Part model, mm, in its own coordinate system. Face numbers are marked on the shaded views. Round coordinates to 2 decimals unless told otherwise and drop trailing zeros. Write each loop counter-clockwise with the first axis right and the second up, starting at its lowest first coordinate (ties: lowest second). Pieces come first, ordered by that corner, then holes. Notation, with made-up numbers: M 13.5,58.25 L 42.5,58.25 A20 cw 42.5,74.25 Z; hole C 57.5,25.25 d7. An arc over 180 degrees is marked long. Use one line per item in the form item = value. Start each with the question number.
Item 1: Probe L1, parallel to X at y = 1.25, z = -4; L2, parallel to X at y = 1, z = -16; L3, parallel to X at y = 2.3, z = -13.25. List the from-to ranges inside material, lowest first.
Item 2: Cut at C-C, the plane z = -16.5. Give the cut face in (x, y).
Item 3: Cut at A-A, the plane x = 30. Give the cut face in (y, z), then the cut area to 3 significant figures.
Item 4: Cut at B-B, the plane z = -5.95. Give the cut face in (x, y).
Item 5: Cut at D-D, the plane y = 1.1. State how many separate pieces and enclosed holes the cut face has, then the cut area to 3 significant figures.
Item 6: Mould opens along Z. For the marked faces 1, 2 and 3 say: +Z half, -Z half, draft (parallel to the pull), parting line (faces both ways), or undercut.
Item 7: Flat gauge pins, fed straight in: pin 1 Ø1.5 at (x, y) = (31, 2) entering from +Z; pin 2 Ø0.9 at (y, z) = (2, -13) entering from -X; pin 3 Ø0.9 at (x, y) = (17, 1.5) entering from -Z; pin 4 Ø1 at (x, z) = (21.5, -1) entering from -Y. Where does each tip first touch, or does it go through?
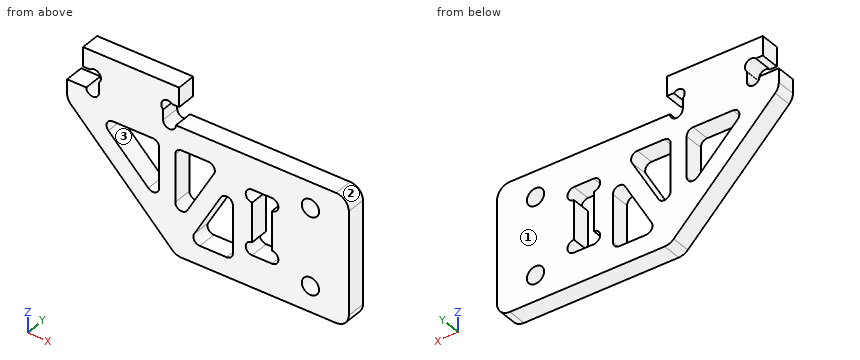
from build123d import *

# Parameters (mm, degrees)
EXTRUDE_1_DEPTH     = 3
SKETCH_2_R          = 1.35
SKETCH_2_W          = 3.1
SKETCH_2_H          = 10.1
CUT_EXTRUDE_1_DEPTH = 49.425200051
SKETCH_5_W          = 15
SKETCH_5_H          = 3
EXTRUDE_2_DEPTH     = 3
SKETCH_3_R          = 1
CUT_EXTRUDE_2_DEPTH = 49.425200051
CUT_EXTRUDE_3_DEPTH = 10
FILLET_1_R          = 1
FILLET_2_R          = 2


with BuildPart() as part:
    # 草图1 → 凸台-拉伸1 (new body)
    with BuildSketch(Plane(origin=(0, 0, 0), x_dir=(1, 0, 0), z_dir=(0, 1, 0))):
        Polygon((0, 0), (5, 0), (5, -3), (15, -3), (15, 0), (44, 0), (44, 20), (17, 20), (0, 3), align=None)
    extrude(amount=EXTRUDE_1_DEPTH)

    # 草图2 → 切除-拉伸1 (cut, through all)
    with BuildSketch(Plane.XZ):
        with Locations(Location((38, -16, 0), (0, 0, 270))):
            Circle(SKETCH_2_R)
        with Locations(Location((38, -4, 0), (0, 0, 90))):
            Circle(SKETCH_2_R)
        with Locations((30.45, -10)):
            Rectangle(SKETCH_2_W, SKETCH_2_H)
    extrude(amount=-CUT_EXTRUDE_1_DEPTH, mode=Mode.SUBTRACT)

    # 草图5 → 凸台-拉伸2 (add)
    with BuildSketch(Plane(origin=(0, 3, 0), x_dir=(1, 0, 0), z_dir=(0, 1, 0))):
        with Locations((10, -4.5)):
            Rectangle(SKETCH_5_W, SKETCH_5_H)
    extrude(amount=-EXTRUDE_2_DEPTH)

    # 草图3 → 切除-拉伸2 (cut, through all)
    with BuildSketch(Plane.XZ):
        with Locations((32, -14.05)):
            Circle(SKETCH_3_R)
        with Locations((16, 0)):
            Circle(SKETCH_3_R)
        with Locations((4, 0)):
            Circle(SKETCH_3_R)
        with Locations((32, -5.95)):
            Circle(SKETCH_3_R)
        with Locations((28.9, -5.95)):
            Circle(SKETCH_3_R)
        with Locations((28.9, -14.05)):
            Circle(SKETCH_3_R)
        with Locations((4.292893219, 2.292893219)):
            Circle(SKETCH_3_R)
        with Locations((15.707106781, 2.292893219)):
            Circle(SKETCH_3_R)
    extrude(amount=-CUT_EXTRUDE_2_DEPTH, mode=Mode.SUBTRACT)

    # 草图4 → 切除-拉伸3 (cut)
    with BuildSketch(Plane(origin=(0, 3, 0), x_dir=(1, 0, 0), z_dir=(0, 1, 0))):
        Polygon((23.789631314, 3.5), (16.896065397, 15.65342471), (16.896065397, 3.5), align=None)
        Polygon((14.396065397, 3.5), (14.396065397, 13.15342471), (4.742640687, 3.5), align=None)
        Polygon((25.9, 4.84657529), (25.9, 17), (19.006434083, 17), align=None)
    extrude(amount=-CUT_EXTRUDE_3_DEPTH, mode=Mode.SUBTRACT)

    # 圆角1
    fillet_1_edges = [part.edges().sort_by_distance(p)[0] for p in [
        (19.006434083, 1.5, -17),
        (25.9, 1.5, -17),
        (25.9, 1.5, -4.84657529),
        (14.396065397, 1.5, -13.15342471),
        (14.396065397, 1.5, -3.5),
        (4.742640687, 1.5, -3.5),
        (16.896065397, 1.5, -15.65342471),
        (23.789631314, 1.5, -3.5),
        (16.896065397, 1.5, -3.5),
    ]]
    fillet(fillet_1_edges, radius=FILLET_1_R)

    # 圆角2
    fillet_2_edges = [part.edges().sort_by_distance(p)[0] for p in [
        (0, 1.5, -3),
        (17, 1.5, -20),
        (44, 1.5, -20),
        (44, 1.5, 0),
    ]]
    fillet(fillet_2_edges, radius=FILLET_2_R)


solid = part.part
Model answer:
q1.L1 = 1 to 6.29, 14.26 to 17.03, 22.94 to 36.65, 39.35 to 44
q1.L2 = 13 to 19.72, 25.9 to 36.65, 39.35 to 44
q1.L3 = 10.25 to 21.13, 25.9 to 28.3, 32.6 to 44
q2.outline = M 13.5,0 L 19.86,0 L 19.86,3 L 13.5,3 Z; M 25.77,0 L 36.75,0 L 36.75,3 L 25.77,3 Z; M 39.25,0 L 44,0 L 44,3 L 39.25,3 Z
q3.outline = M 0,-20 L 3,-20 L 3,-15.05 L 0,-15.05 Z; M 0,-4.95 L 3,-4.95 L 3,0 L 0,0 Z
q3.area = 29.7 mm²
q4.outline = M 2.95,0 L 7.19,0 L 7.19,3 L 2.95,3 Z; M 14.4,0 L 16.9,0 L 16.9,3 L 14.4,3 Z; M 22.4,0 L 27.9,0 L 27.9,3 L 22.4,3 Z; M 33,0 L 44,0 L 44,3 L 33,3 Z
q5.separate_pieces = 1
q5.enclosed_holes = 6
q5.area = 634 mm²
q6.face_1 = draft
q6.face_2 = +Z half
q6.face_3 = undercut
q7.pin_1 = 0
q7.pin_2 = 9.55
q7.pin_3 = -19.96
q7.pin_4 = 0
